Read the model definition and answer for the solid it produces. Units are mm, in the model's axes. A direction names the side the tool comes from. Coordinates: 2 decimals unless noted, no trailing zeros. Loops run counter-clockwise (first coordinate to the right, second up) from the corner with the lowest first, then second, coordinate; pieces in that order, holes last.
Q1. The mould has two halves that part along X. Classify faces 1 (the face through (-840, 292, -449)), 2 (the face through (-1042, 130, 0)), 3 (the face through (-952.625, 231.699, -49.3)): pulls with the +X half, pulls with the -X half, needs draft (parallel to the pull), parting line crosses it, or undercut.
Q2. Straight lines are drawn through the part: line 1 (Y direction, x = -1045, z = -21.5); line 2 (X direction, y = 48, z = -280); line 3 (Z direction, x = -220, y = 35). For each, find the intervals that lie inside material, in ascending order.
Q3. Which of the six approach directions +Z, -Z, +X, -X, +Y, -Y give full straight-line access (tool end or side, diameter ignored) to faces 4 (the face through (-857, 183, -500)), 5 (the face through (-299.357, 54.23, -219.152)), 6 (the face through (-1048, 375, -100)), 7 (the face through (-647.34, 54.23, -121.68)), 8 (the face through (-840, 292, -49))?
Q4. Section D-D (y = 413.5) is taken. Give the vertices of the cut face in (x, z), then the cut area to 3 significant figures.
Q5. Flat-ended cylindrical pins translate along their axes: P1, Ø10, axis at y = 392, z = -409.5, coming from the +X side; P2, Ø8, axis at x = -704, z = -280.5, coming from the +Y side. Find the tip coordinate at first contact, or state that the pin passes through.
Q6. Section B-B (x = -985) is taken. Give the vertices of the cut face in (y, z).
Q7. Section C-C (z = -120) is taken. Give the vertices of the cut face in (x, y).
Q8. Section A-A (y = 270) is taken. Give the vertices of the cut face in (x, z).
from build123d import *

# Parameters (mm, degrees)
SKETCH1_R           = 100
BOSS_EXTRUDE1_DEPTH = 110
SKETCH2_W           = 410
SKETCH2_H           = 100
BOSS_EXTRUDE2_DEPTH = 370
SKETCH3_R           = 100
CUT_EXTRUDE1_DEPTH  = 501


with BuildPart() as part:
    # Sketch1 → Boss-Extrude1 (new body)
    with BuildSketch(Plane(origin=(0, 0, 0), x_dir=(1, 0, 0), z_dir=(0, 1, 0))):
        with BuildLine():
            Line((-460, 0), (-460, 240))
            Line((-460, 240), (-840, 0))
            Line((-840, 0), (-1250, 0))
            Line((-1250, 0), (-1250, 500))
            Line((-1250, 500), (-220, 500))
            ThreePointArc((-220, 500), (-64.436508139, 435.563491861), (0, 280))
            Line((0, 280), (0, 0))
            Line((0, 0), (-460, 0))
        make_face()
        with Locations((-220, 280)):
            Circle(SKETCH1_R, mode=Mode.SUBTRACT)
    extrude(amount=BOSS_EXTRUDE1_DEPTH)

    # Sketch2 → Boss-Extrude2 (add)
    with BuildSketch(Plane(origin=(0, 110, 0), x_dir=(1, 0, 0), z_dir=(0, 1, 0))):
        with Locations((-1045, 450)):
            Rectangle(SKETCH2_W, SKETCH2_H)
        with Locations((-1045, 50)):
            Rectangle(SKETCH2_W, SKETCH2_H)
    extrude(amount=BOSS_EXTRUDE2_DEPTH)

    # Sketch3 → Cut-Extrude1 (cut, through all)
    with BuildSketch(Plane.XY):
        with Locations((-1045, 270)):
            Circle(SKETCH3_R)
    extrude(amount=-CUT_EXTRUDE1_DEPTH, mode=Mode.SUBTRACT)


solid = part.part
Numbers:
1. face 1: pulls with the +X half
1. face 2: needs draft
1. face 3: undercut
2. line 1: y = 0 to 170, 370 to 480
2. line 2: x = -1250 to -320, -120 to 0
2. line 3: z = -500 to -380, -180 to 0
3. face 4: -Z, +X, -X, +Y, -Y
3. face 5: +Y, -Y
3. face 6: +X, -X, +Y
3. face 7: +Z, +Y, -Y
3. face 8: +Z, -Z, +X, +Y
4. outline: (-1250, -500) - (-840, -500) - (-840, -400) - (-1250, -400) - close; (-1250, -100) - (-840, -100) - (-840, 0) - (-1250, 0) - close
4. area: 82,000 mm2
5. P1: stops at x = -840
5. P2: stops at y = 110
6. outline: (0, -500) - (190, -500) - (190, -400) - (110, -400) - (110, -100) - (190, -100) - (190, 0) - (0, 0) - close; (350, -500) - (480, -500) - (480, -400) - (350, -400) - close; (350, -100) - (480, -100) - (480, 0) - (350, 0) - close
7. outline: (-1250, 0) - (-650, 0) - (-650, 110) - (-1250, 110) - close; (-460, 0) - (0, 0) - (0, 110) - (-460, 110) - close
8. outline: (-1250, -500) - (-1145, -500) - (-1145, -400) - (-1250, -400) - close; (-1250, -100) - (-1145, -100) - (-1145, 0) - (-1250, 0) - close; (-945, -500) - (-840, -500) - (-840, -400) - (-945, -400) - close; (-945, -100) - (-840, -100) - (-840, 0) - (-945, 0) - close
